from build123d import *

# Parameters (mm, degrees)
SKETCH_1_W               = 27
SKETCH_1_H               = 15
EXTRUDE_1_DEPTH          = 11
CUT_EXTRUDE_6_DEPTH      = 16
SKETCH_2_OUTSIDE_W       = 35.558
SKETCH_2_OUTSIDE_H       = 23.558
SKETCH_2_OUTSIDE_W_2     = 28.581712044
SKETCH_2_OUTSIDE_H_2     = 12
CUT_EXTRUDE_1_DEPTH      = 10.4
CUT_EXTRUDE_1_DEPTH_BACK = 0.7
SKETCH_6_W               = 5
SKETCH_6_H               = 12
EXTRUDE_2_DEPTH          = 3.803863
SKETCH_7_R               = 0.8
CUT_EXTRUDE_7_DEPTH      = 14.5


with BuildPart() as part:
    # Эскиз1 → Бобышка-Вытянуть1 (new body)
    with BuildSketch(Plane.XY):
        with Locations((13.5, 7.5)):
            Rectangle(SKETCH_1_W, SKETCH_1_H)
    extrude(amount=EXTRUDE_1_DEPTH)

    # Эскиз5 → Вырез-Вытянуть6 (cut, through all)
    with BuildSketch(Plane(origin=(0, 15, 0), x_dir=(1, 0, 0), z_dir=(0, 1, 0))):
        Polygon((0, 0), (0, -8.886908691), (4.14403358, 0), align=None)
        Polygon((27, -11), (27, -1.6), (8.914830922, -1.6), (4.531538935, -11), align=None)
        Polygon((0, -11), (4.531538935, -11), (0, -8.886908691), align=None)
        Polygon((23.997690311, 0), (27, -1.4), (27, 0), align=None)
    extrude(amount=-CUT_EXTRUDE_6_DEPTH, mode=Mode.SUBTRACT)

    # Эскиз2 outside → Вырез-Вытянуть1 (cut, two sides)
    with BuildSketch(Plane.XY.offset(1.6)) as cut_extrude_1_sk:
        with Locations((13.5, 7.5)):
            Rectangle(SKETCH_2_OUTSIDE_W, SKETCH_2_OUTSIDE_H)
        with Locations((13.459567245, 7.5)):
            Rectangle(SKETCH_2_OUTSIDE_W_2, SKETCH_2_OUTSIDE_H_2, mode=Mode.SUBTRACT)
    extrude(amount=CUT_EXTRUDE_1_DEPTH, mode=Mode.SUBTRACT)
    extrude(cut_extrude_1_sk.sketch, amount=-CUT_EXTRUDE_1_DEPTH_BACK, mode=Mode.SUBTRACT)

    # Эскиз6 → Бобышка-Вытянуть2 (add)
    with BuildSketch(Plane(origin=(-3.40388351, 0, 7.299651743), x_dir=(0.906307787, 0, 0.422618262), z_dir=(-0.422618262, 0, 0.906307787))):
        with Locations((6.255769903, 7.5)):
            Rectangle(SKETCH_6_W, SKETCH_6_H)
    extrude(amount=EXTRUDE_2_DEPTH)

    # Эскиз7 → Вырез-Вытянуть7 (cut, through all)
    with BuildSketch(Plane(origin=(0, 13.5, 0), x_dir=(1, 0, 0), z_dir=(0, 1, 0))):
        with Locations((4.598685766, -5.298008566)):
            Circle(SKETCH_7_R)
    extrude(amount=-CUT_EXTRUDE_7_DEPTH, mode=Mode.SUBTRACT)


solid = part.part
CAD build for the part. Positions are in the model's coordinates, mm. A direction names the side the tool comes from. Round coordinates to 2 decimals unless told otherwise and drop trailing zeros. Loops run counter-clockwise (first coordinate to the right, second up) from the corner with the lowest first, then second, coordinate; pieces in that order, holes last. Notation, with made-up numbers: M -36.5,30.5 L 17.5,30.5 A26 ccw 17.5,65.5 Z; hole C -25.75,37.5 d4. An arc over 180 degrees is marked long. One line per question, with ' | ' between items. Start each with the question number.
Item 1: Cut at B-B, the plane y = 4. Write the cut outline in (x, z), plus the area to 3 significant figures.
Item 2: Cut at A-A, the plane x = 13.5. Write the cut outline in (y, z), plus the area to 3 significant figures.
Item 3: Two-plate mould, pull along X, no slides. Class faces 5 (the flat face through (0.626, 7.584, 13.376)), 6 (the flat face through (25.5, 7.6, 0.7)), 7 (the cylindrical face through (5.029, 7.584, 4.623)), 8 (the flat face through (15, 1, 0.9)): pulls with the +X half, pulls with the -X half, needs draft (parallel to the pull), parting line crosses it, or undercut.
Item 4: Cut at D-D, the plane x = 7.75. Write the cut outline in (y, z), plus the area to 3 significant figures.
Item 5: Pin check, flat tips, straight feed: pin 1 Ø1.2 at (x, y) = (10.5, 14) entering from +Z; pin 2 Ø1.5 at (y, z) = (13, 5.5) entering from -X; pin 3 Ø1.4 at (x, z) = (4.6, 5.3) entering from -Y; pin 4 Ø0.8 at (x, y) = (11, 1) entering from +Z. Stop position of each tip, or through.
Item 6: Which spindle directions (+Z, -Z, +X, -X, +Y, -Y) get a long thin tool onto all of the face, cutting with end or side? Do faces 1 (the flat face through (15, 14, 0.9)), 2 (the flat face through (18, 8, 1.6)), 3 (the flat face through (5.22, 1.5, 6.02)), 4 (the flat face through (14.7, 0, 0.4)). Say none if no direction does.
Item 7: Wall check: line 1 (Z direction, x = 18, y = 8); line 2 (Z direction, x = 4.5, y = 11); line 3 (Z direction, x = 20.75, y = 1.25). Give the ranges that are in metal, low to high.
Item 8: Cut at C-C, the plane z = 8.25. Write the cut outline in (x, y).
Responses:
1) outline: M -1.61,12.33 L 4.14,0 L 24,0 L 27,1.4 L 27,1.6 L 8.91,1.6 L 2.92,14.45 Z; hole C 4.6,5.3 d1.6 | area: 98.1 mm²
2) outline: M 0,0 L 15,0 L 15,0.9 L 13.5,0.9 L 13.5,1.6 L 1.5,1.6 L 1.5,0.9 L 0,0.9 Z | area: 21.9 mm²
3) face 5: pulls with the -X half | face 6: pulls with the +X half | face 7: undercut | face 8: needs draft
4) outline: M 0,0 L 15,0 L 15,0.9 L 13.5,0.9 L 13.5,4.1 L 1.5,4.1 L 1.5,0.9 L 0,0.9 Z | area: 51.9 mm²
5) pin 1: stops at z = 1.6 | pin 2: stops at x = 1.23 | pin 3: passes through | pin 4: stops at z = 0.9
6) face 1: +Z, +X, -X, +Y | face 2: +Z, +X, +Y, -Y | face 3: +Z, +X, -X, -Y | face 4: +Z, -Z, +X, -X, -Y
7) line 1: z = 0 to 1.6 | line 2: z = 0 to 4.5, 6.09 to 11.07 | line 3: z = 0 to 0.9
8) outline: M 0.3,1.5 L 5.81,1.5 L 5.81,13.5 L 0.3,13.5 Z
